Can you work these out from the drawing? Everything is in mm from the part's minimum corner. Coordinates: 2 decimals unless noted, no trailing zeros. Order: outer loops, then holes, each group sorted by start corner. A loop starts at its lowest first (then second) coordinate and runs counter-clockwise, first axis right, second up. Notation, with made-up numbers: M 36,69 L 84,69 A24 ccw 84,105 Z; hole C 30.25,44 d4. An arc over 180 degrees is marked long. Answer as a JSON object with one key per item and string values.
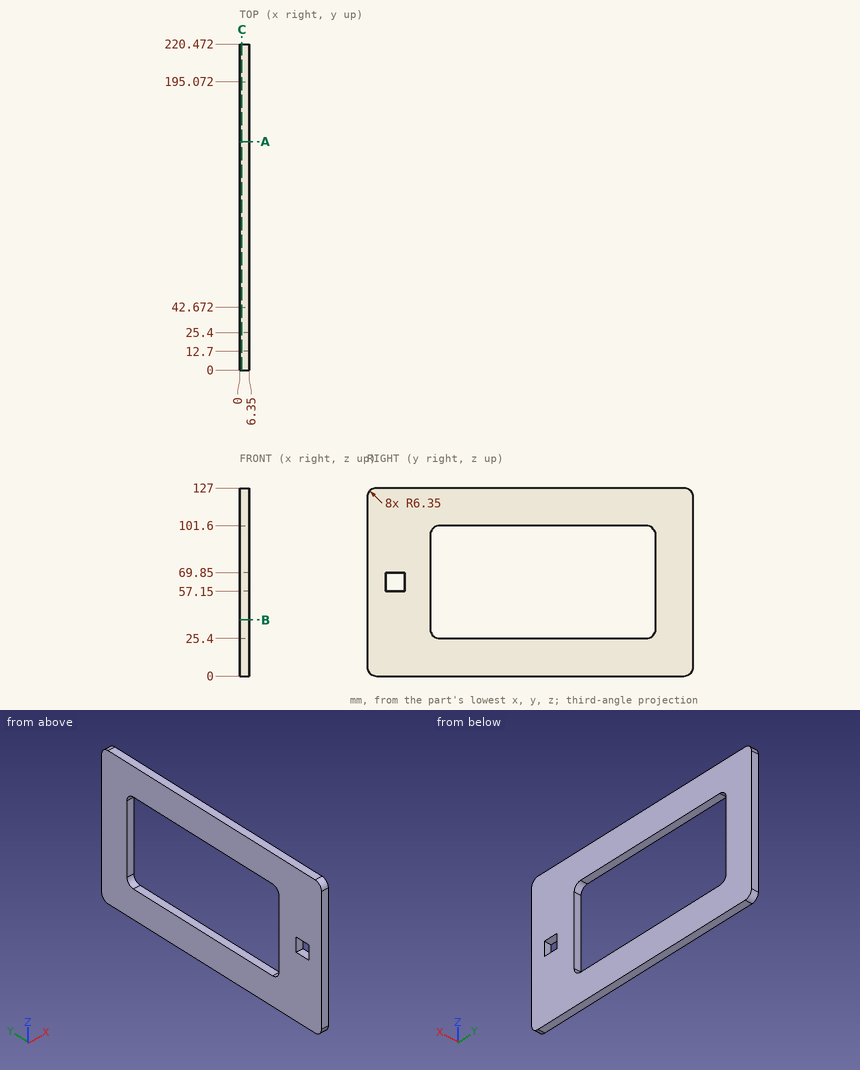
Item 1: I want a section at B-B, the plane z = 38. Write out the boundary of the cut face in (x, y), plus the area to 3 significant figures.
Answers follow:
{"outline": "M 0,0 L 6.35,0 L 6.35,42.67 L 0,42.67 Z; M 0,195.07 L 6.35,195.07 L 6.35,220.47 L 0,220.47 Z", "area": "432 mm^2"}
Item 2: Please list where these lines run through material, in increasing order: line 1 (Y direction, x = 2.25, z = 69.5); line 2 (Y direction, x = 1, z = 72); line 3 (Z direction, x = 0.5, y = 161.5).
Answers follow:
{"line 1": "y = 0 to 12.7, 25.4 to 42.67, 195.07 to 220.47", "line 2": "y = 0 to 42.67, 195.07 to 220.47", "line 3": "z = 0 to 25.4, 101.6 to 127"}
Item 3: I want a section at C-C, the plane x = 1.5. Write out the boundary of the cut face in (y, z).
Answers follow:
{"outline": "M 0,6.35 A6.35 ccw 6.35,0 L 214.12,0 A6.35 ccw 220.47,6.35 L 220.47,120.65 A6.35 ccw 214.12,127 L 6.35,127 A6.35 ccw 0,120.65 Z; hole M 12.7,57.15 L 25.4,57.15 L 25.4,69.85 L 12.7,69.85 Z; hole M 42.67,31.75 A6.35 ccw 49.02,25.4 L 188.72,25.4 A6.35 ccw 195.07,31.75 L 195.07,95.25 A6.35 ccw 188.72,101.6 L 49.02,101.6 A6.35 ccw 42.67,95.25 Z"}
Item 4: I want a section at A-A, the plane y = 154.5. Write out the boundary of the cut face in (x, z).
Answers follow:
{"outline": "M 0,0 L 6.35,0 L 6.35,25.4 L 0,25.4 Z; M 0,101.6 L 6.35,101.6 L 6.35,127 L 0,127 Z"}
